Read the model definition and answer for the solid it produces. Units are mm, in the model's axes. A direction names the side the tool comes from. Coordinates: 2 decimals unless noted, no trailing zeros. Loops run counter-clockwise (first coordinate to the right, second up) from the corner with the lowest first, then second, coordinate; pieces in that order, holes last. Notation, with made-up numbers: (2.5, -2) -> (53.5, -2) arc R19 ccw to (53.5, 8) -> close; hole circle Ø2 at (82.25, -33). An arc over 180 degrees is marked (long way). Answer as a JSON object with one key per item and string values. Group by question number.
1) Which of the six approach directions +Z, -Z, +X, -X, +Y, -Y give full straight-line access (tool end or side, diameter ignored) to faces 4 (the face through (10, 49, -85)), 5 (the face through (-137, 67, -5)), 6 (the face through (-30, 29, -27)), 7 (the face through (33, 49, -15)), 8 (the face through (-60, 14, -27))?
2) Section D-D, the plane y = 85 is taken. Give the vertices of the cut face in (x, z).
3) Section C-C, the plane z = -45 is taken. Give the vertices of the cut face in (x, y), plus the area to 3 significant figures.
4) Section A-A, the plane y = 50 is taken. Give the vertices of the cut face in (x, z), plus the area to 4 significant figures.
5) Consider probe 1 along Y at (x, z) = (-78, -4.75); probe 2 along Y at (x, z) = (-137.5, -9.75); probe 3 along X at (y, z) = (85, -16.3). Determine where each line is inside the solid, lowest interval first. Write a range as [from, to].
6) Determine the mould class of faces 1 (the face through (-160, 49, -10)), 2 (the face through (-140.27, 65.85, -12.6)), 3 (the face through (-59, 49, 0)) for opening direction X: released by +X, released by -X, zero draft, split by the parting line, or undercut.
7) Flat-ended cylindrical pins translate along their axes: P1, Ø16.5, axis at y = 83, z = -26.5, coming from the -X side; P2, Ø12, axis at y = 26, z = -44, coming from the +X side; P3, Ø3, axis at y = 28.5, z = -42.5, coming from the -X side; P4, Ø5, axis at x = -105, y = 90, coming from the -Z side. Find the tip coordinate at first contact, or state that the pin passes through.
8) Section B-B, the plane x = 32.5 is taken. Give the vertices of the cut face in (y, z).
from build123d import *

# Parameters (mm, degrees)
BOSS_EXTRUDE2_DEPTH = 100
SKETCH3_W           = 60
SKETCH3_H           = 29
BOSS_EXTRUDE3_DEPTH = 15
SKETCH4_R           = 4
CUT_EXTRUDE1_DEPTH  = 15
HOLE2_AT_2_COUNT    = 2
HOLE2_AT_2_PITCH    = 70
SKETCH9_R           = 3
CUT_EXTRUDE2_DEPTH  = 15
SKETCH10_R          = 9
CUT_EXTRUDE3_DEPTH  = 52


with BuildPart() as part:
    # Sketch1 → Boss-Extrude2 (new body)
    with BuildSketch(Plane(origin=(0, 0, 0), x_dir=(1, 0, 0), z_dir=(0, 1, 0))):
        Polygon((-160, 0), (45, 0), (45, 15), (20, 15), (20, 85), (0, 85), (0, 20), (-160, 20), align=None)
    extrude(amount=BOSS_EXTRUDE2_DEPTH)

    # Sketch3 → Boss-Extrude3 (add)
    with BuildSketch(Plane(origin=(0, 0, -20), x_dir=(-1, 0, 0), z_dir=(0, 0, -1))):
        with Locations((30, 85.5)):
            Rectangle(SKETCH3_W, SKETCH3_H)
        with Locations((30, 14.5)):
            Rectangle(SKETCH3_W, SKETCH3_H)
    extrude(amount=BOSS_EXTRUDE3_DEPTH)

    # Sketch4 → Cut-Extrude1 (cut)
    with BuildSketch(Plane(origin=(0, 0, -15), x_dir=(-1, 0, 0), z_dir=(0, 0, -1))):
        with Locations((-32.5, 85)):
            Circle(SKETCH4_R)
        with Locations((-32.5, 15)):
            Circle(SKETCH4_R)
    extrude(amount=-CUT_EXTRUDE1_DEPTH, mode=Mode.SUBTRACT)

    # Sketch8 → Hole2 (revolve, cut)
    with BuildSketch(Plane(origin=(-78, 85, -20), x_dir=(0, 1, 0), z_dir=(1, 0, 0))):
        Polygon((0, 0), (0, 20), (4, 20), (4, 7.103012167), (7.5, 5), (7.5, 0), align=None)
    hole2 = revolve(axis=Axis((-78, 85, -26.130023899), (0, 0, 1)), mode=Mode.SUBTRACT)

    # Hole2 at 2: Hole2 ×2
    with Locations(*[(0, -i * HOLE2_AT_2_PITCH, 0) for i in range(1, HOLE2_AT_2_COUNT)]):
        add(hole2, mode=Mode.SUBTRACT)

    # Sketch9 → Cut-Extrude2 (cut)
    with BuildSketch(Plane(origin=(0, 0, -20), x_dir=(-1, 0, 0), z_dir=(0, 0, -1))):
        with Locations((137.5, 67)):
            Circle(SKETCH9_R)
        with Locations((137.5, 33)):
            Circle(SKETCH9_R)
    extrude(amount=-CUT_EXTRUDE2_DEPTH, mode=Mode.SUBTRACT)

    # Sketch10 → Cut-Extrude3 (cut)
    with BuildSketch(Plane(origin=(20, 0, 0), x_dir=(0, 0, -1), z_dir=(1, 0, 0))):
        with Locations((45, 50)):
            Circle(SKETCH10_R)
    extrude(amount=-CUT_EXTRUDE3_DEPTH, mode=Mode.SUBTRACT)


solid = part.part
Determined:
{
 "1": {"face 4": "-Z, +X, -X, +Y, -Y", "face 5": "-Z", "face 6": "-Z, -X", "face 7": "-Z, +X, +Y, -Y", "face 8": "-Z, -X, +Y, -Y"},
 "2": {"outline": "(-160, -20) -> (-85.5, -20) -> (-85.5, -15) -> (-82, -12.9) -> (-82, 0) -> (-160, 0) -> close; (-74, -12.9) -> (-70.5, -15) -> (-70.5, -20) -> (-60, -20) -> (-60, -35) -> (0, -35) -> (0, -85) -> (20, -85) -> (20, -15) -> (28.5, -15) -> (28.5, 0) -> (-74, 0) -> close; (36.5, -15) -> (45, -15) -> (45, 0) -> (36.5, 0) -> close"},
 "3": {"outline": "(0, 0) -> (20, 0) -> (20, 41) -> (0, 41) -> close; (0, 59) -> (20, 59) -> (20, 100) -> (0, 100) -> close", "area": "1,640 mm²"},
 "4": {"outline": "(-160, -20) -> (0, -20) -> (0, -36) -> (20, -36) -> (20, -15) -> (45, -15) -> (45, 0) -> (-160, 0) -> close; (0, -85) -> (20, -85) -> (20, -54) -> (0, -54) -> close", "area": "4,915 mm²"},
 "5": {"probe 1": "[0, 11], [19, 81], [89, 100]", "probe 2": "[0, 30], [36, 64], [70, 100]", "probe 3": "[-160, -85.5], [-70.5, 20]"},
 "6": {"face 1": "released by -X", "face 2": "undercut", "face 3": "zero draft"},
 "7": {"P1": "x = -160", "P2": "x = 20", "P3": "x = 0", "P4": "z = -20"},
 "8": {"outline": "(0, -15) -> (11, -15) -> (11, 0) -> (0, 0) -> close; (19, -15) -> (81, -15) -> (81, 0) -> (19, 0) -> close; (89, -15) -> (100, -15) -> (100, 0) -> (89, 0) -> close"}
}
